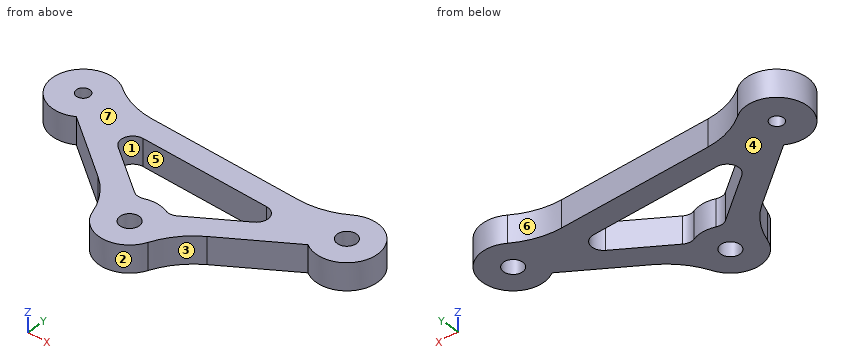
from build123d import *

# Parameters (mm, degrees)
SKETCH2_R             = 8
SKETCH2_R_2           = 1.75
BOSS_EXTRUDE2_DEPTH   = 7
SKETCH2_R_3           = 2.5
BOSS_EXTRUDE2_2_DEPTH = 7
BOSS_EXTRUDE2_3_DEPTH = 7
BOSS_EXTRUDE3_DEPTH   = 7
FILLET4_R             = 3
FILLET5_R             = 20
FILLET6_R             = 20


with BuildPart() as part:
    # Sketch2 → Boss-Extrude2 (new body)
    with BuildSketch(Plane.XY):
        with Locations((-75.824618394, 230.884392152)):
            Circle(SKETCH2_R)
        with Locations((-75.824618394, 230.884392152)):
            Circle(SKETCH2_R_2, mode=Mode.SUBTRACT)
    extrude(amount=BOSS_EXTRUDE2_DEPTH)



with BuildPart() as body_2:
    # Sketch2 → Boss-Extrude2 2 (new body)
    with BuildSketch(Plane.XY):
        with Locations((-4.277553922, 228.026598272)):
            Circle(SKETCH2_R)
        with Locations((-4.277553922, 228.026598272)):
            Circle(SKETCH2_R_3, mode=Mode.SUBTRACT)
    extrude(amount=BOSS_EXTRUDE2_2_DEPTH)


with BuildPart() as body_3:
    # Sketch2 → Boss-Extrude2 3 (new body)
    with BuildSketch(Plane.XY):
        with Locations((-41.051610566, 204.406598272)):
            Circle(SKETCH2_R)
        with Locations((-41.051610566, 204.406598272)):
            Circle(SKETCH2_R_3, mode=Mode.SUBTRACT)
    extrude(amount=BOSS_EXTRUDE2_3_DEPTH)


with BuildPart() as part_1:
    add(part.part)

    add(body_2.part)  # Boss-Extrude3 merges body 2

    add(body_3.part)  # Boss-Extrude3 merges body 3
    # Sketch2_6 → Boss-Extrude3 (add)
    with BuildSketch(Plane.XY):
        with BuildLine():
            Line((-13.90449039, 225.408733387), (-12.138758245, 226.542864268))
            ThreePointArc((-12.138758245, 226.542864268), (-12.2560646, 227.440622708), (-12.271179822, 228.345886496))
            Line((-12.271179822, 228.345886496), (-67.830992493, 230.565103927))
            ThreePointArc((-67.830992493, 230.565103927), (-67.918262005, 229.663929677), (-68.106798475, 228.778387472))
            Line((-68.106798475, 228.778387472), (-66.437148094, 227.507037612))
            Line((-66.437148094, 227.507037612), (-13.90449039, 225.408733387))
        make_face()
        with BuildLine():
            Line((-67.830992493, 230.565103927), (-12.271179822, 228.345886496))
            ThreePointArc((-12.271179822, 228.345886496), (-12.063001048, 229.866927876), (-11.568110377, 231.32019609))
            Line((-11.568110377, 231.32019609), (-68.294595771, 233.586013758))
            ThreePointArc((-68.294595771, 233.586013758), (-67.942988455, 232.255490073), (-67.824618394, 230.884392152))
            ThreePointArc((-67.824618394, 230.884392152), (-67.826212077, 230.72471623), (-67.830992493, 230.565103927))
        make_face()
        with BuildLine():
            Line((-11.008685122, 223.703188417), (-34.320479367, 208.730008128))
            ThreePointArc((-34.320479367, 208.730008128), (-33.618575942, 207.364637533), (-33.190406244, 205.890332276))
            Line((-33.190406244, 205.890332276), (-8.896200854, 221.494515869))
            ThreePointArc((-8.896200854, 221.494515869), (-10.058896717, 222.497034502), (-11.008685122, 223.703188417))
        make_face()
        with BuildLine():
            ThreePointArc((-36.432963635, 210.938680676), (-35.270267772, 209.936162043), (-34.320479367, 208.730008128))
            Line((-34.320479367, 208.730008128), (-11.008685122, 223.703188417))
            ThreePointArc((-11.008685122, 223.703188417), (-11.710588547, 225.068559011), (-12.138758245, 226.542864268))
            Line((-12.138758245, 226.542864268), (-13.90449039, 225.408733387))
            Line((-13.90449039, 225.408733387), (-36.432963635, 210.938680676))
        make_face()
        with BuildLine():
            ThreePointArc((-47.416469362, 209.253099331), (-46.373505799, 210.379657047), (-45.134554691, 211.286247048))
            Line((-45.134554691, 211.286247048), (-66.437148094, 227.507037612))
            Line((-66.437148094, 227.507037612), (-68.106798475, 228.778387472))
            ThreePointArc((-68.106798475, 228.778387472), (-68.651192431, 227.342929183), (-69.459759598, 226.037891093))
            Line((-69.459759598, 226.037891093), (-47.416469362, 209.253099331))
        make_face()
        with BuildLine():
            Line((-71.741674269, 224.004743376), (-48.769430485, 206.512602952))
            ThreePointArc((-48.769430485, 206.512602952), (-48.225036529, 207.948061241), (-47.416469362, 209.253099331))
            Line((-47.416469362, 209.253099331), (-69.459759598, 226.037891093))
            ThreePointArc((-69.459759598, 226.037891093), (-70.502723161, 224.911333377), (-71.741674269, 224.004743376))
        make_face()
    extrude(amount=BOSS_EXTRUDE3_DEPTH)

    # Fillet4
    fillet4_edges = [part_1.edges().sort_by_distance(p)[0] for p in [
        (-45.134554691, 211.286247048, 3.5),
        (-66.437148094, 227.507037612, 3.5),
        (-13.90449039, 225.408733387, 3.5),
        (-36.432963635, 210.938680676, 3.5),
    ]]
    fillet(fillet4_edges, radius=FILLET4_R)

    # Fillet5
    fillet5_edges = [part_1.edges().sort_by_distance(p)[0] for p in [
        (-11.568110377, 231.32019609, 3.5),
        (-68.294595771, 233.586013758, 3.5),
    ]]
    fillet(fillet5_edges, radius=FILLET5_R)

    # Fillet6
    fillet6_edges = [part_1.edges().sort_by_distance(p)[0] for p in [
        (-48.769430485, 206.512602952, 3.5),
        (-33.190406244, 205.890332276, 3.5),
    ]]
    fillet(fillet6_edges, radius=FILLET6_R)


solid = part_1.part
Source: CAD feature listing. Evaluate the final solid. Frame: model axes, mm. Face numbers are marked on the shaded views. A direction names the side the tool comes from. Give positions to 0.01 mm unless a question says otherwise; leave off trailing zeros. Order: outer loops, then holes, each group sorted by start corner. A loop starts at its lowest first (then second) coordinate and runs counter-clockwise, first axis right, second up. Notation, with made-up numbers: (-20.5, 9) -> (7.5, 9) arc R23 cw to (7.5, 35) -> close; hole circle Ø11 at (23.5, 23). An arc over 180 degrees is marked (long way). Write item = value, one per line.
Item 1: Section query D-D (x = -10). Output: boundary loops of the cut face in (y, z).
Check result:
outline = (220.79, 0) -> (233.95, 0) -> (233.95, 7) -> (220.79, 7) -> close
Item 2: Set-up query: the marked faces 5, 6 and 7. Return all of +Z, -Z, +X, -X, +Y, -Y with unobstructed straight access to the full face (end or side cutting, diameter ignored); none if empty.
Check result:
face_5 = +Z, -Z
face_6 = +Z, -Z, +Y
face_7 = +Z, +X, -X, +Y, -Y
Item 3: Contact query for flat-ended pins moving along their axis: pin 1 (4 mm diameter, centred on x = -68.5, z = 4, fed in from +Y); pin 2 (4 mm diameter, centred on y = 209, z = 3.5, fed in from -X); pin 3 (1 mm diameter, centred on x = -44.5, z = 3, fed in from -Y). Output: stop coordinate, or through.
Check result:
pin_1 = 236.9
pin_2 = -54.71
pin_3 = 196.97
Item 4: Section query B-B (y = 217). Output: boundary loops of the cut face in (x, z), then the cut area to 3 significant figures.
Check result:
outline = (-62.54, 0) -> (-52.64, 0) -> (-52.64, 7) -> (-62.54, 7) -> close; (-27, 0) -> (-15.89, 0) -> (-15.89, 7) -> (-27, 7) -> close
area = 147 mm²
Item 5: Mould query, pull axis X, two halves, no side actions, for the marked faces 1, 2, 3 and 4. Classes: +X half, -X half, draft (parallel to the pull), parting line (faces both ways), or undercut.
Check result:
face_1 = undercut
face_2 = parting line
face_3 = +X half
face_4 = draft
Item 6: Ray query, probe 1 along X at (y, z) = (221, 6); probe 2 along Y at (x, z) = (-56, 5); probe 3 along Y at (x, z) = (-44, 2.5). Return the intervals inside material, ascending.
Check result:
probe_1 = -67.8 to -57.89, -21.12 to -9.67, -8.1 to -0.45
probe_2 = 212.02 to 219.56, 227.09 to 233.09
probe_3 = 196.97 to 211.86, 226.61 to 232.62
Item 7: Section query A-A (x = -75). Output: boundary loops of the cut face in (y, z), then the cut area to 3 significant figures.
Check result:
outline = (222.93, 0) -> (229.34, 0) -> (229.34, 7) -> (222.93, 7) -> close; (232.43, 0) -> (238.84, 0) -> (238.84, 7) -> (232.43, 7) -> close
area = 89.8 mm²
Item 8: Section query C-C (z = 4). Output: boundary loops of the cut face in (x, y).
Check result:
outline = (-71.74, 224) -> (-55.57, 211.69) arc R20 cw to (-48.66, 201.94) arc R8 ccw to (-33.66, 201.34) arc R20 cw to (-25.99, 210.51) -> (-8.9, 221.49) arc R8 ccw (long way) to (-8.57, 234.77) arc R20 cw to (-20.11, 231.66) -> (-59.75, 233.24) arc R20 cw to (-71, 237.27) arc R8 ccw (long way) to start; hole circle Ø3.5 at (-75.82, 230.88); hole (-58.87, 221.74) -> (-46.57, 212.38) arc R3 ccw to (-43.74, 211.94) arc R8 cw to (-37.77, 211.7) arc R3 ccw to (-34.92, 211.91) -> (-21.91, 220.27) arc R3 ccw to (-23.41, 225.79) -> (-56.93, 227.13) arc R3 ccw to start; hole circle Ø5 at (-41.05, 204.41); hole circle Ø5 at (-4.28, 228.03)
